The model under review builds one solid part; all positions refer to its coordinate system, in mm. Give positions to 0.01 mm unless a question says otherwise; leave off trailing zeros. Loops run counter-clockwise (first coordinate to the right, second up) from the corner with the lowest first, then second, coordinate; pieces in that order, holes last. Notation, with made-up numbers: (0.5, 21) -> (20.5, 21) arc R23 cw to (20.5, 48) -> close; hole circle Ø4 at (27, 45). An arc over 180 degrees is marked (long way). Write each question's results on one line, items separated by ' | '. Start each with the question number.
Q1. We need section B-B (x = 5). Write out the cut boundary in (y, z).
Q2. Wall thickness on L1, parallel to X at y = -12, z = 75; L2, parallel to Y at x = -3.75, z = 167; L3, parallel to Z at x = 11.5, y = -0.5: over which ranges is each line inside the solid? List them lowest first. Write a range as [from, to].
Q3. We need section A-A (y = 2.5). Write out the cut boundary in (x, z), plus the area to 3 significant figures.
Q4. We need section C-C (z = 104). Write out the cut boundary in (x, y), plus the area to 3 significant figures.
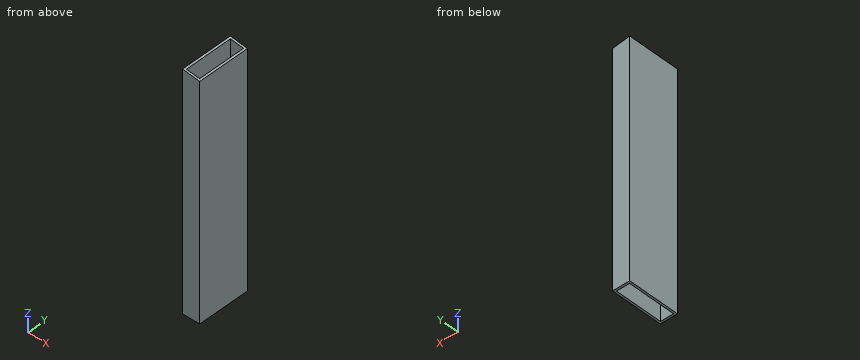
from build123d import *

# Parameters (mm, degrees)
SKETCH2_W               = 9.652
SKETCH2_H               = 3.048
SKETCH2_W_2             = 3.048
SKETCH2_H_2             = 35.052
BOSS_EXTRUDE1_DEPTH     = 343
SKETCH3_W               = 25.4
SKETCH3_H               = 76.2
SKETCH3_W_2             = 19.304
SKETCH3_H_2             = 70.104
BOSS_EXTRUDE2_DEPTH     = 50
CUT_EXTRUDE2_DEPTH      = 1
CUT_EXTRUDE2_DEPTH_BACK = 77.2


with BuildPart() as part:
    # Sketch2 → Boss-Extrude1 (new body)
    with BuildSketch(Plane.XY):
        Polygon((-12.7, 0), (-9.652, 0), (-9.652, 35.052), (-9.652, 38.1), (-12.7, 38.1), align=None)
        with Locations((-4.826, 36.576)):
            Rectangle(SKETCH2_W, SKETCH2_H)
        Polygon((0, 38.1), (0, 35.052), (9.652, 35.052), (9.652, 0), (12.7, 0), (12.7, 38.1), align=None)
        with Locations((11.176, -17.526)):
            Rectangle(SKETCH2_W_2, SKETCH2_H_2)
        Polygon((-9.652, -35.052), (-9.652, 0), (-12.7, 0), (-12.7, -38.1), (0, -38.1), (0, -35.052), align=None)
        Polygon((9.652, -35.052), (0, -35.052), (0, -38.1), (12.7, -38.1), (12.7, -35.052), align=None)
    extrude(amount=BOSS_EXTRUDE1_DEPTH)

    # Sketch3 → Boss-Extrude2 (add)
    with BuildSketch(Plane.XY.offset(343)):
        Rectangle(SKETCH3_W, SKETCH3_H)
        Rectangle(SKETCH3_W_2, SKETCH3_H_2, mode=Mode.SUBTRACT)
    extrude(amount=BOSS_EXTRUDE2_DEPTH)

    # Sketch5 → Cut-Extrude2 (cut, two sides)
    with BuildSketch(Plane(origin=(0, 38.1, 0), x_dir=(1, 0, 0), z_dir=(0, 1, 0))) as cut_extrude2_sk:
        Polygon((12.7, -391.250668344), (12.534006261, -391.403498707), (0, -343), (-12.7, -344.617644511), (-12.7, -393), (12.7, -393), align=None)
        Polygon((12.7, -341.382355489), (12.7, -391.250668344), (75.559800862, -333.375677395), align=None)
        Polygon((0, -343), (12.534006261, -391.403498707), (12.7, -391.250668344), (12.7, -341.382355489), align=None)
    extrude(amount=CUT_EXTRUDE2_DEPTH, mode=Mode.SUBTRACT)
    extrude(cut_extrude2_sk.sketch, amount=-CUT_EXTRUDE2_DEPTH_BACK, mode=Mode.SUBTRACT)


solid = part.part
Output:
1) outline: (-38.1, 0) -> (-35.05, 0) -> (-35.05, 342.36) -> (-38.1, 342.36) -> close; (35.05, 0) -> (38.1, 0) -> (38.1, 342.36) -> (35.05, 342.36) -> close
2) L1: [-12.7, -9.65], [9.65, 12.7] | L2: [-38.1, -35.05], [35.05, 38.1] | L3: [0, 341.54]
3) outline: (-12.7, 0) -> (-9.65, 0) -> (-9.65, 344.23) -> (-12.7, 344.62) -> close; (9.65, 0) -> (12.7, 0) -> (12.7, 341.38) -> (9.65, 341.77) -> close | area: 2,090 mm2
4) outline: (-12.7, -38.1) -> (12.7, -38.1) -> (12.7, 38.1) -> (-12.7, 38.1) -> close; hole (-9.65, -35.05) -> (9.65, -35.05) -> (9.65, 35.05) -> (-9.65, 35.05) -> close | area: 582 mm2
